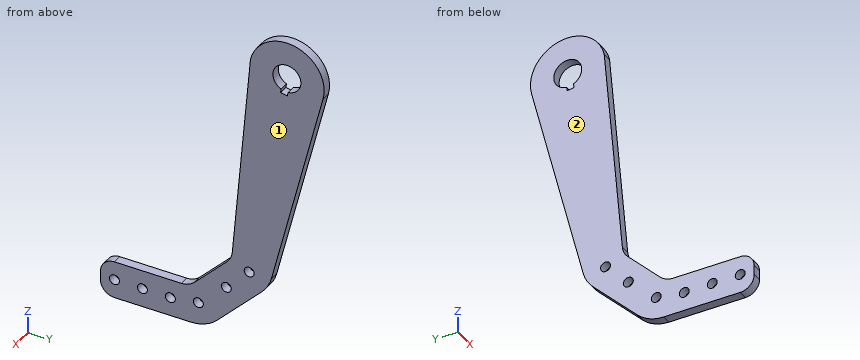
from build123d import *

# Parameters (mm, degrees)
SKETCH1_R                   = 19.05
BOSS_EXTRUDE1_DEPTH         = 12.7
FILLET1_R                   = 25.4
FILLET2_R                   = 50.8
F_1_2_CLEARANCE_HOLE1_D     = 13.49248
F_1_2_CLEARANCE_HOLE1_DEPTH = 38.1
F_1_2_CLEARANCE_HOLE1_TIP   = 4.053549943
FILLET3_R                   = 19.05
CUT_EXTRUDE1_DEPTH          = 13.7
F_1_2_CLEARANCE_HOLE2_D     = 13.49248


with BuildPart() as part:
    # Sketch1 → Boss-Extrude1 (new body)
    with BuildSketch(Plane(origin=(0, 0, 0), x_dir=(0, 0, -1), z_dir=(1, 0, 0))):
        with BuildLine():
            Line((390.630407277, -109.766978243), (305.29908743, -24.435658396))
            Line((305.29908743, -24.435658396), (12.395871839, 49.264412727))
            ThreePointArc((12.395871839, 49.264412727), (-49.470959365, 11.544010545), (-10.688712274, -49.662777107))
            Line((-10.688712274, -49.662777107), (281.610658396, -75.235658396))
            Line((281.610658396, -75.235658396), (339.725, -133.35))
            Line((339.725, -133.35), (339.725, -254))
            Line((339.725, -254), (390.630407277, -254))
            Line((390.630407277, -254), (390.630407277, -109.766978243))
        make_face()
        Circle(SKETCH1_R, mode=Mode.SUBTRACT)
    extrude(amount=BOSS_EXTRUDE1_DEPTH)

    # Fillet1
    fillet1_edges = [part.edges().sort_by_distance(p)[0] for p in [
        (6.35, -133.35, -339.725),
        (6.35, -75.235658396, -281.610658396),
    ]]
    fillet(fillet1_edges, radius=FILLET1_R)

    # Fillet2
    fillet2_edges = [part.edges().sort_by_distance(p)[0] for p in [
        (6.35, -24.435658396, -305.29908743),
        (6.35, -109.766978243, -390.630407277),
    ]]
    fillet(fillet2_edges, radius=FILLET2_R)

    # 1/2 Clearance Hole1
    with Locations(Plane(origin=(12.7, 0, 0), x_dir=(0, 0, -1), z_dir=(1, 0, 0))):
        with Locations((365.125, -234.95), (365.125, -196.85), (365.125, -158.75), (359.5071206, -120.65), (324.846024484, -82.55)):
            Hole(F_1_2_CLEARANCE_HOLE1_D / 2, depth=F_1_2_CLEARANCE_HOLE1_DEPTH)
            with Locations((0, 0, -(F_1_2_CLEARANCE_HOLE1_DEPTH + F_1_2_CLEARANCE_HOLE1_TIP / 2))):  # 118° drill point
                Cone(0, F_1_2_CLEARANCE_HOLE1_D / 2, F_1_2_CLEARANCE_HOLE1_TIP, mode=Mode.SUBTRACT)

    # Fillet3
    fillet3_edges = [part.edges().sort_by_distance(p)[0] for p in [
        (6.35, -254, -390.630407277),
        (6.35, -254, -339.725),
    ]]
    fillet(fillet3_edges, radius=FILLET3_R)

    # Sketch4 → Cut-Extrude1 (cut, through all)
    with BuildSketch(Plane(origin=(12.7, 0, 0), x_dir=(0, 0, -1), z_dir=(1, 0, 0))):
        Polygon((23.478806451, -3.972505995), (24.27330765, 0.723255295), (14.88178507, 2.312257693), (13.292782672, -7.079264887), (22.684305252, -8.668267285), align=None)
    extrude(amount=-CUT_EXTRUDE1_DEPTH, mode=Mode.SUBTRACT)

    # 1/2 Clearance Hole2 (through all)
    with Locations(Plane(origin=(12.7, 0, 0), x_dir=(0, 0, -1), z_dir=(1, 0, 0))):
        with Locations((292.641331438, -51.40137192)):
            Hole(F_1_2_CLEARANCE_HOLE2_D / 2)


solid = part.part
Geometry check sheet. Reference: the model listing, model coordinates, mm. Face numbers are marked on the shaded views. Round coordinates to 2 decimals unless told otherwise and drop trailing zeros. Write each loop counter-clockwise with the first axis right and the second up, starting at its lowest first coordinate (ties: lowest second). Pieces come first, ordered by that corner, then holes.
Item 1: Section check B-B (z = 0). Record the boundary of the cut face in (x, y), plus the area to 3 significant figures.
Determined:
outline: (0, -50.6) - (12.7, -50.6) - (12.7, -19.05) - (0, -19.05) - close; (0, 19.05) - (12.7, 19.05) - (12.7, 50.8) - (0, 50.8) - close
area: 804 mm2
Item 2: Material ranges on line 1 along Y through (x, z) = (10.75, -289) (1 decimal); line 2 along Y through (x, z) = (8.5, -287.5); line 3 along Z through (x, y) = (9.5, -178.5) (3 decimals), recorded low to high.
Determined:
line 1: y = -82.6 to -57.1, -45.7 to -20.3
line 2: y = -81.15 to -55.77, -47.03 to -19.96
line 3: z = -390.63 to -339.725
Item 3: Mould release check, pull along X, two halves, no side actions. Record for the marked faces 1 and 2: +X half, -X half, draft (parallel to the pull), parting line (faces both ways), or undercut.
Determined:
face 1: +X half
face 2: -X half
Item 4: Section check D-D (z = -252). Record the boundary of the cut face in (x, y), plus the area to 3 significant figures.
Determined:
outline: (0, -72.65) - (12.7, -72.65) - (12.7, -11.02) - (0, -11.02) - close
area: 783 mm2
Item 5: Go/stop test with flat-tipped pins: pin 1 Ø2 at (x, z) = (10, -237.5) entering from -Y; pin 2 Ø2 at (x, z) = (11, -176) entering from -Y; pin 3 Ø1.5 at (x, z) = (11, -312.5) entering from -Y (3 decimals). Record where each tip stops, or that it passes through.
Determined:
pin 1: stops at y = -71.46
pin 2: stops at y = -66.08
pin 3: stops at y = -106.875
Item 6: Section check C-C (x = 6.25). Record the boundary of the cut face in (y, z) (3 decimals), plus the area to 3 significant figures.
Determined:
outline: (-254, -371.58) arc R19.05 ccw to (-234.95, -390.63) - (-130.809, -390.63) arc R50.8 ccw to (-94.888, -375.751) - (-34.356, -315.219) arc R50.8 ccw to (-21.012, -291.694) - (49.264, -12.396) arc R50.8 ccw (long way) to (-49.663, 10.689) - (-74.43, -272.401) arc R25.4 cw to (-81.773, -288.148) - (-125.911, -332.286) arc R25.4 cw to (-143.871, -339.725) - (-234.95, -339.725) arc R19.05 ccw to (-254, -358.775) - close; hole circle Ø13.492 at (-234.95, -365.125); hole circle Ø13.492 at (-196.85, -365.125); hole circle Ø13.492 at (-158.75, -365.125); hole circle Ø13.492 at (-120.65, -359.507); hole circle Ø13.492 at (-82.55, -324.846); hole circle Ø13.492 at (-51.401, -292.641); hole (-8.668, -22.684) - (0.723, -24.273) - (1.619, -18.981) arc R19.05 ccw (long way) to (-7.773, -17.392) - close
area: 37,000 mm2
Item 7: Section check A-A (y = -158.75). Record the boundary of the cut face in (x, z) (3 decimals), plus the area to 3 significant figures.
Determined:
outline: (0, -390.63) - (12.7, -390.63) - (12.7, -371.871) - (0, -371.871) - close; (0, -358.379) - (12.7, -358.379) - (12.7, -339.725) - (0, -339.725) - close
area: 475 mm2
